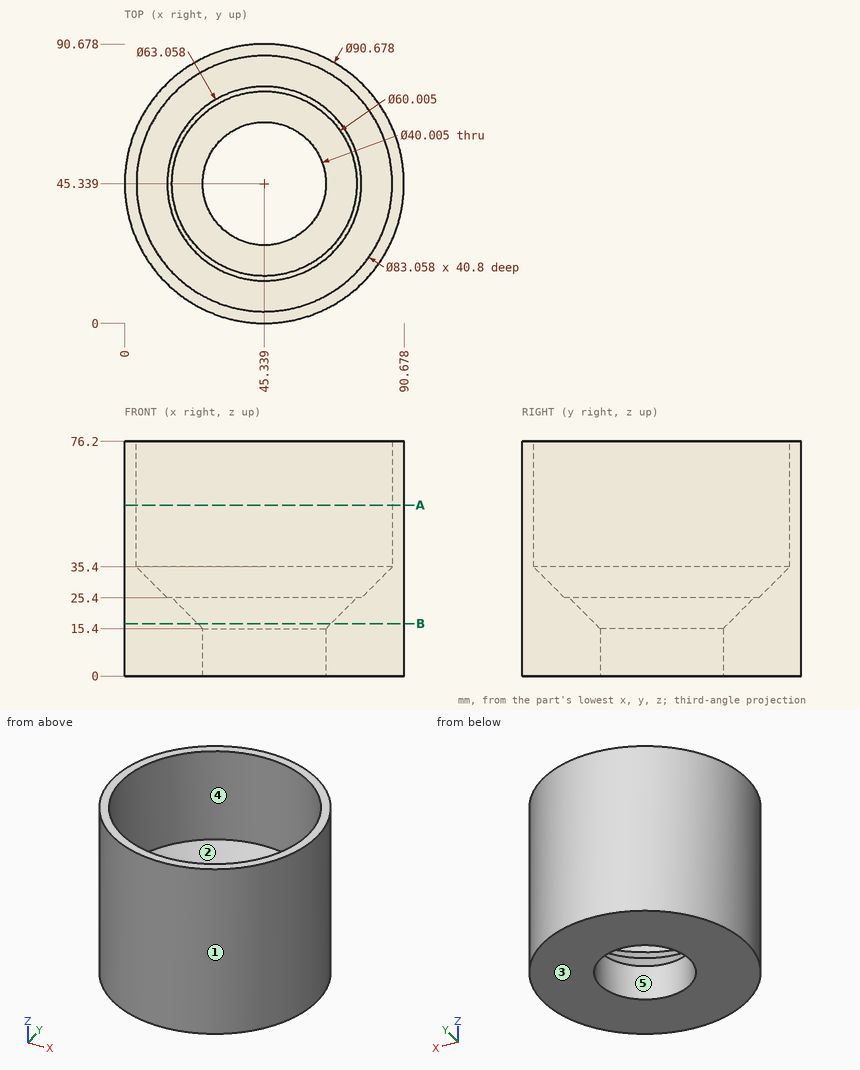
Answer from the drawing. Dimensions are ordinates in mm from the lowest x, y and z of the part. A direction names the side the tool comes from. Round coordinates to 2 decimals unless told otherwise and drop trailing zeros. Loops run counter-clockwise (first coordinate to the right, second up) from the corner with the lowest first, then second, coordinate; pieces in that order, holes last.
Q1. Which of the six approach directions +Z, -Z, +X, -X, +Y, -Y give full straight-line access (tool end or side, diameter ignored) to the marked faces 4 and 5?
Q2. Section A-A on z = 55.5 is taken. Write down the section's boundary in (x, y).
Q3. Each of these flat-tipped pins is pushed along its axis until it touches: pin 1 (8 mm diameter, centred on y = 67.5, z = 14, fed in from +X); pin 2 (4 mm diameter, centred on x = 69.5, y = 59.5, fed in from -Z); pin 3 (12 mm diameter, centred on x = 79.5, z = 45.5, fed in from -Y); pin 4 (2 mm diameter, centred on x = 77, z = 39.5, fed in from +Y). Where does it stop, or does it pass through?
Q4. Determine the mould class of the marked faces 1, 2 and 3 for opening direction X: released by +X, released by -X, zero draft, split by the parting line, or undercut.
Q5. Consider probe 1 along X at (y, z) = (46.5, 50); probe 2 along Y at (x, z) = (28, 54); probe 3 along Y at (x, z) = (79, 68). Determine where each line is inside the solid, lowest interval first.
Q6. Section B-B on z = 17 is taken. Write down the section's boundary in (x, y) (1 decimal).
Output:
1. face 4: +Z
1. face 5: +Z, -Z
2. outline: circle Ø90.68 at (45.34, 45.34); hole circle Ø83.06 at (45.34, 45.34)
3. pin 1: stops at x = 86.88
3. pin 2: stops at z = 0
3. pin 3: stops at y = 9.81
3. pin 4: stops at y = 78.74
4. face 1: split by the parting line
4. face 2: undercut
4. face 3: zero draft
5. probe 1: x = 0.01 to 3.83, 86.85 to 90.66
5. probe 2: y = 3.45 to 7.6, 83.08 to 87.23
5. probe 3: y = 14.97 to 21.02, 69.66 to 75.71
6. outline: circle Ø90.7 at (45.3, 45.3); hole circle Ø43.2 at (45.3, 45.3)
